```python
from build123d import *

# Parameters (mm, degrees)
ESQUISSE1_R             = 3.75
EXTRUSION1_DEPTH        = 25.5
ESQUISSE2_R             = 2.5
EXTRUSION2_DEPTH        = 10.5
ESQUISSE3_R             = 1.5
ENL_V_MAT_EXTRU_1_DEPTH = 8
ESQUISSE5_W             = 3.097754454
ESQUISSE5_H             = 3
ESQUISSE6_W             = 5.14619883
ESQUISSE6_H             = 0.986249407
ENL_V_MAT_EXTRU_3_DEPTH = 2
ESQUISSE8_OUTSIDE_W     = 17.006
ESQUISSE8_OUTSIDE_H     = 17.006
ESQUISSE8_OUTSIDE_R     = 2.5
EXTRUSION5_DEPTH        = 15.5
CHANFREIN1_SIZE         = 0.5


with BuildPart() as part:
    # Esquisse1 → Extrusion1 (new body)
    with BuildSketch(Plane.XY):
        Circle(ESQUISSE1_R)
    extrude(amount=EXTRUSION1_DEPTH)

    # Esquisse2 → Extrusion2 (add)
    with BuildSketch(Plane(origin=(0, 0, 0), x_dir=(-1, 0, 0), z_dir=(0, 0, -1))):
        with Locations(Location((0, 0, 0), (0, 0, 180))):
            Circle(ESQUISSE2_R)
    extrude(amount=EXTRUSION2_DEPTH)

    # Esquisse3 → Enlèv. mat.-Extru.1 (cut)
    with BuildSketch(Plane.XY.offset(25.5)):
        Circle(ESQUISSE3_R)
    extrude(amount=-ENL_V_MAT_EXTRU_1_DEPTH, mode=Mode.SUBTRACT)

    # Esquisse5 → Enlèvement de matière-Révolution1 (revolve, cut)
    with BuildSketch(Plane(origin=(0, 0, 0), x_dir=(1, 0, 0), z_dir=(0, 1, 0))):
        with Locations((3.548877227, 5.25)):
            Rectangle(ESQUISSE5_W, ESQUISSE5_H)
    revolve(axis=Axis((0, 0, -10.5), (0, 0, 1)), mode=Mode.SUBTRACT)

    # Esquisse6 → Enlèv. mat.-Extru.3 (cut)
    with BuildSketch(Plane(origin=(0, 0, -10.5), x_dir=(-1, 0, 0), z_dir=(0, 0, -1))):
        with Locations((0.031610558, -2.493124704)):
            Rectangle(ESQUISSE6_W, ESQUISSE6_H)
    extrude(amount=-ENL_V_MAT_EXTRU_3_DEPTH, mode=Mode.SUBTRACT)

    # Esquisse8 outside → Extrusion5 (cut)
    with BuildSketch(Plane(origin=(0, 0, 0), x_dir=(-1, 0, 0), z_dir=(0, 0, -1))):
        Rectangle(ESQUISSE8_OUTSIDE_W, ESQUISSE8_OUTSIDE_H)
        with Locations(Location((0, 0, 0), (0, 0, 180))):
            Circle(ESQUISSE8_OUTSIDE_R, mode=Mode.SUBTRACT)
    extrude(amount=-EXTRUSION5_DEPTH, mode=Mode.SUBTRACT)

    # Chanfrein1
    chanfrein1_edges = [part.edges().sort_by_distance(p)[0] for p in [
        (-3.75, 0, 25.5),
    ]]
    chamfer(chanfrein1_edges, length=CHANFREIN1_SIZE)


solid = part.part
```
Here's how the part is built. I have some questions about the finished solid (model axes, mm). A direction names the side the tool comes from. Round coordinates to 2 decimals unless told otherwise and drop trailing zeros. Write each loop counter-clockwise with the first axis right and the second up, starting at its lowest first coordinate (ties: lowest second). Pieces come first, ordered by that corner, then holes.
Q1. If we section it at B-B on x = 0: Write out the boundary of the cut face in (y, z).
Q2. If we mould it in two halves opening along X, with no side actions, what happens to faces 1 (the flat face through (0, 3, 15.5)), 2 (the cylindrical face through (-3.746, 0.165, 20.184)), 3 (the flat face through (0, 0, 17.5))? For each: +X half, -X half, draft (parallel to the pull), parting line (faces both ways), or undercut.
Q3. Please list where these lines run through material, in increasing order: probe 1 along Y at (x, z) = (0, 20.5); probe 2 along Z at (x, y) = (1, 2); probe 3 along Z at (x, y) = (1, -2.5).
Q4. If we section it at C-C on z = 1.5: Write out the boundary of the cut face in (x, y).
Q5. Will these pins go through, and if not, where does the flat tip stop? P1, Ø2, axis at x = -1.5, z = 0, coming from the -Y side; P2, Ø3, axis at x = 1, z = 1.5, coming from the +Y side; P3, Ø1.5, axis at x = -2.5, z = 12.5, coming from the +Y side.
Q6. If we section it at A-A on y = 0: Write out the boundary of the cut face in (x, z), plus the area to 3 significant figures.
Q7. Which directions (+Z, -Z, +X, -X, +Y, -Y) give clear straight access to the entire face, cutting with the end or side of a thin tool? Please do faces 4 (the cylindrical face through (-1.5, 0.07, 21.56)), 5 (the cylindrical face through (-0.54, 2.44, -8.6)), 6 (the cylindrical face through (0, -2, -5)), 7 (the flat face through (0, -2, -10)).
Answer below:
1. outline: (-3.75, 15.5) - (-2.5, 15.5) - (-2.5, -3.75) - (-2, -3.75) - (-2, -6.75) - (-2.5, -6.75) - (-2.5, -8.5) - (-2, -8.5) - (-2, -10.5) - (2.5, -10.5) - (2.5, -6.75) - (2, -6.75) - (2, -3.75) - (2.5, -3.75) - (2.5, 15.5) - (3.75, 15.5) - (3.75, 25) - (3.25, 25.5) - (1.5, 25.5) - (1.5, 17.5) - (-1.5, 17.5) - (-1.5, 25.5) - (-3.25, 25.5) - (-3.75, 25) - close
2. face 1: draft
2. face 2: parting line
2. face 3: undercut
3. probe 1: y = -3.75 to -1.5, 1.5 to 3.75
3. probe 2: z = -10.5 to -6.75, -3.75 to 25.5
3. probe 3: z = 15.5 to 25.5
4. outline: circle Ø5 at (0, 0)
5. P1: stops at y = -2.45
5. P2: stops at y = 2.5
5. P3: stops at y = 1.79
6. outline: (-3.75, 15.5) - (-2.5, 15.5) - (-2.5, -3.75) - (-2, -3.75) - (-2, -6.75) - (-2.5, -6.75) - (-2.5, -10.5) - (2.5, -10.5) - (2.5, -6.75) - (2, -6.75) - (2, -3.75) - (2.5, -3.75) - (2.5, 15.5) - (3.75, 15.5) - (3.75, 25) - (3.25, 25.5) - (1.5, 25.5) - (1.5, 17.5) - (-1.5, 17.5) - (-1.5, 25.5) - (-3.25, 25.5) - (-3.75, 25) - close
6. area: 178 mm2
7. face 4: +Z
7. face 5: -Z
7. face 6: none
7. face 7: -Z, +X, -X, -Y
